Input: part model. Units: mm. Frame: model coordinates. Face numbers are marked on the shaded views. A direction names the side the tool comes from. Give positions to 0.01 mm unless a question says otherwise; leave off trailing zeros. Order: outer loops, then holes, each group sorted by start corner. A loop starts at its lowest first (then second) coordinate and runs counter-clockwise, first axis right, second up. Notation, with made-up numbers: (40.5, 5) - (99.5, 5) arc R20 ccw to (99.5, 16) - close; hole circle Ø8 at (35.5, 70.25). An arc over 180 degrees is marked (long way). Answer in a Markdown table with one row per item. Add a question column.
Autodesk Inventor part; units mm, degrees
ref_plane "YZ Plane" through (0, 0, 0) normal (1, 0, 0) x (0, 1, 0)
ref_plane "XZ Plane" through (0, 0, 0) normal (0, 1, 0) x (-1, 0, 0)
ref_plane "XY Plane" through (0, 0, 0) normal (0, 0, 1) x (1, 0, 0)
sketch "Sketch1" plane through (0, 0, 0) normal (1, 0, 0) x (0, 1, 0)
  line L0 (0, 0) -> (0, -21.5)
  line L1 (0, -21.5) -> (4, -21.5)
  line L2 (4, -21.5) -> (4, -10.5)
  line L3 (4, -10.5) -> (3, -10.5)
  line L4 (3, -10.5) -> (3, -1.5)
  line L5 (3, -1.5) -> (2.85, -1.5)
  line L6 (2.85, -1.5) -> (2.85, -0.7)
  line L7 (2.85, -0.7) -> (3, -0.7)
  line L8 (3, -0.7) -> (3, -0.15)
  line L9 (3, -0.15) -> (2.85, 0)
  line L10 (2.85, 0) -> (0, 0)
  dimension "d0" = 21.5
  dimension "d1" = 0.15
  dimension "d2" = 0.15
  dimension "d3" = 0.7
  dimension "d4" = 0.15
  dimension "d5" = 0.8
  dimension "d6" = 11
  dimension "d7" = 9
  dimension "d8" = 4
  dimension "d9" = 3
revolve "Revolution1" add sketch "Sketch1" angle 360 about axis through (0, 0, 0) along (0, 0, -1)
properties part number "Component 3 (Planet Gear Axis)"
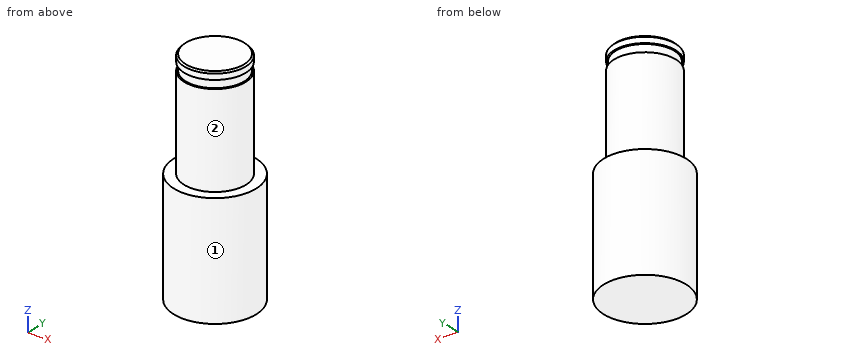
Q1. Access query for the marked faces 1 and 2. Directions: +Z, -Z, +X, -X, +Y, -Y. A direction counts if a zero-diameter tool reaches every point of the face in a straight line with its end or side. Return the directions, or none.
Q2. Line query: probe 1 along Z at (x, y) = (-0.75, -3); probe 2 along X at (y, z) = (0, -5.5); probe 3 along X at (y, z) = (1.5, -11.25). Output: solid intervals per line, ascending.
Q3. Section C-C, the plane z = -15.5. Return loops of the section in (x, y), then the cut area to 3 significant figures.
Q4. Section D-D, the plane z = -10. Return loops of the section in (x, y), then the cut area to 3 significant figures.
Q5. Contact query for flat-ended pins moving along their axis: P1, Ø3, axis at x = -2.5, z = -3, coming from the +Y side; P2, Ø4, axis at y = 2.5, z = -15.5, coming from the +X side; P3, Ø1, axis at x = -2.5, z = -9, coming from the +Y side; P4, Ø2, axis at x = 2.5, y = -1, coming from the +Z side. Output: stop coordinate, or through.
Q6. Section A-A, the plane y = 0. Return loops of the section in (x, z), then the cut area to 3 significant figures.
Computed:
| question | item | result |
|---|---|---|
| 1 | face 1 | +Z, -Z |
| 1 | face 2 | +Z |
| 2 | probe 1 | z = -21.5 to -10.5 |
| 2 | probe 2 | x = -3 to 3 |
| 2 | probe 3 | x = -3.71 to 3.71 |
| 3 | outline | circle Ø8 at (0, 0) |
| 3 | area | 50.3 mm^2 |
| 4 | outline | circle Ø6 at (0, 0) |
| 4 | area | 28.3 mm^2 |
| 5 | P1 | stops at y = 2.83 |
| 5 | P2 | stops at x = 3.97 |
| 5 | P3 | stops at y = 2.24 |
| 5 | P4 | stops at z = 0 |
| 6 | outline | (-4, -21.5) - (4, -21.5) - (4, -10.5) - (3, -10.5) - (3, -1.5) - (2.85, -1.5) - (2.85, -0.7) - (3, -0.7) - (3, -0.15) - (2.85, 0) - (-2.85, 0) - (-3, -0.15) - (-3, -0.7) - (-2.85, -0.7) - (-2.85, -1.5) - (-3, -1.5) - (-3, -10.5) - (-4, -10.5) - close |
| 6 | area | 151 mm^2 |
